The model under review builds one solid part; all positions refer to its coordinate system, in mm. A direction names the side the tool comes from. Give positions to 0.01 mm unless a question says otherwise; leave off trailing zeros. Order: outer loops, then holes, each group sorted by start corner. A loop starts at its lowest first (then second) coordinate and runs counter-clockwise, first axis right, second up. Notation, with made-up numbers: (-38.5, 71.5) - (-21.5, 71.5) arc R9 ccw to (-21.5, 75.5) - close; hole circle Ø6 at (42.5, 7.5). An arc over 180 degrees is marked (long way). Write item = value, one per line. Start each with the question number.
1. Machinability: for faces 1 (the flat face through (0.095, -31.284, 3.372)), 2 (the cylindrical face through (-7.493, 0.33, 3.451)), 3 (the cylindrical face through (-12.5, -0.1, 8)), which of the approach directions +Z, -Z, +X, -X, +Y, -Y give a long, thin tool a straight path to every point of the face, cutting with its end or side? Answer none if there is none.
2. Wall thickness on probe 1 along Y at (x, z) = (0, 3); probe 2 along Y at (x, z) = (0, 2.5); probe 3 along Z at (x, y) = (7, 10): over which ranges is each line inside the solid? List them lowest first.
3. We need section D-D, the plane y = 31. Give the boundary of the cut face in (x, z).
4. For P1, Ø7.5, axis at x = -6, y = 11.5, coming from the -Z side; P2, Ø6, axis at x = 1, z = 1, coming from the -Y side; P3, Ø8, axis at x = -9.5, y = -16.5, coming from the +Z side; P4, Ø1, axis at x = 2.5, z = 10.5, coming from the -Y side, all flat-tipped, find the tip position at first contact; note any pin that passes through.
5. Mouldability with a two-part tool opening along Y and no side actions: class faces 4 (the flat face through (-5.4, -5.2, 9)), 5 (the flat face through (2, 6, 0)), 6 (the flat face through (0.028, 41.947, 17.646)) as pulls with the +Y half, pulls with the -Y half, needs draft (parallel to the pull), parting line crosses it, or undercut.
6. We need section B-B, the plane y = 0. Give the boundary of the cut face in (x, z), and give its area (3 significant figures).
7. We need section A-A, the plane x = 0. Give the boundary of the cut face in (y, z).
8. We need section C-C, the plane z = 2.25. Give the boundary of the cut face in (x, y) (3 decimals), and give its area (3 significant figures).
from build123d import *

# Parameters (mm, degrees)
ESQUISSE1_R          = 7.5
ESQUISSE1_R_2        = 6
BASE_EXTRUSION_DEPTH = 7
ESQUISSE2_R          = 6
BOSS_EXTRU_1_DEPTH   = 2
CONG_1_R             = 1
BOSS_EXTRU_2_DEPTH   = 2
BOSS_EXTRU_3_DEPTH   = 2


with BuildPart() as part:
    # Esquisse1 → Base-Extrusion (new body)
    with BuildSketch(Plane.XY):
        Circle(ESQUISSE1_R)
        Circle(ESQUISSE1_R_2, mode=Mode.SUBTRACT)
    extrude(amount=BASE_EXTRUSION_DEPTH)

    # Esquisse2 → Boss.-Extru.1 (add)
    with BuildSketch(Plane.XY.offset(7)):
        with BuildLine():
            Line((-7, 25), (7, 25))
            Line((7, 25), (10, 7.5))
            ThreePointArc((10, 7.5), (12.5, 0), (10, -7.5))
            Line((10, -7.5), (7, -25))
            Line((7, -25), (-7, -25))
            Line((-7, -25), (-10, -7.5))
            ThreePointArc((-10, -7.5), (-12.5, 0), (-10, 7.5))
            Line((-10, 7.5), (-7, 25))
        make_face()
        Circle(ESQUISSE2_R, mode=Mode.SUBTRACT)
    extrude(amount=BOSS_EXTRU_1_DEPTH)

    # Congé1
    cong_1_edges = [part.edges().sort_by_distance(p)[0] for p in [
        (-6, 0, 9),
    ]]
    fillet(cong_1_edges, radius=CONG_1_R)

    # Esquisse3 → Boss.-Extru.2 (add)
    with BuildSketch(Plane(origin=(0, 2.352885683, -4.075317547), x_dir=(-1, 0, 0), z_dir=(0, 0.499999999999998, -0.8660254037844398))):
        Polygon((-7, 25.150635095), (-2, 45.150635095), (2, 45.150635095), (7, 25.150635095), align=None)
    extrude(amount=BOSS_EXTRU_2_DEPTH)

    # Esquisse4 → Boss.-Extru.3 (add)
    with BuildSketch(Plane(origin=(0, -9.281088913, 16.075317547), x_dir=(1, 0, 0), z_dir=(0, -0.49999999999999806, 0.8660254037844398))):
        Polygon((-7, -17.150635095), (7, -17.150635095), (2, -37.150635095), (-2, -37.150635095), align=None)
    extrude(amount=BOSS_EXTRU_3_DEPTH)


solid = part.part
Model answer:
q1.face_1 = -Z, +X, -X
q1.face_2 = -Z
q1.face_3 = +Z, -Z, -X
q2.probe_1 = -35.93 to -31.93, -7.5 to -6, 6 to 7.5
q2.probe_2 = -36.79 to -32.79, -7.5 to -6, 6 to 7.5
q2.probe_3 = 7 to 9
q3.outline = (-5.31, 10.15) - (5.31, 10.15) - (5.02, 12.46) - (-5.02, 12.46) - close
q4.P1 = 7
q4.P2 = -42.45
q4.P3 = 9
q4.P4 = 26.73
q5.face_4 = undercut
q5.face_5 = needs draft
q5.face_6 = pulls with the +Y half
q6.outline = (-12.5, 7) - (-7.5, 7) - (-7.5, 0) - (-6, 0) - (-6, 8) arc R1 ccw to (-7, 9) - (-12.5, 9) - close; (6, 0) - (7.5, 0) - (7.5, 7) - (12.5, 7) - (12.5, 9) - (7, 9) arc R1 ccw to (6, 8) - close
q6.area = 46.6 mm2
q7.outline = (-42.45, -0.77) - (-41.45, -2.5) - (-25, 7) - (-7.5, 7) - (-7.5, 0) - (-6, 0) - (-6, 8) arc R1 ccw to (-7, 9) - (-25, 9) - (-25.13, 9.23) - close; (6, 0) - (7.5, 0) - (7.5, 7) - (25, 7) - (25.13, 6.77) - (42.45, 16.77) - (41.45, 18.5) - (25, 9) - (7, 9) arc R1 ccw to (6, 8) - close
q8.outline = circle Ø15 at (0, 0); (-4.375, -33.227) - (-3.509, -37.227) - (3.509, -37.227) - (4.375, -33.227) - close; hole circle Ø12 at (0, 0)
q8.area = 95.2 mm2
